```python
from build123d import *

# Parameters (mm, degrees)
SKETCH1_R           = 2.6
BOSS_EXTRUDE3_DEPTH = 10
SKETCH5_R           = 5
CUT_EXTRUDE3_DEPTH  = 20
FILLET2_R           = 1


with BuildPart() as part:
    # Sketch1 → Boss-Extrude3 (new body)
    with BuildSketch(Plane(origin=(0, 0, 0), x_dir=(1, 0, 0), z_dir=(0, 1, 0))):
        with BuildLine():
            Line((-13.5, -10), (13.5, -10))
            ThreePointArc((13.5, -10), (15.621320344, -9.121320344), (16.5, -7))
            Line((16.5, -7), (16.5, 7))
            ThreePointArc((16.5, 7), (15.621320344, 9.121320344), (13.5, 10))
            Line((13.5, 10), (-13.5, 10))
            ThreePointArc((-13.5, 10), (-15.621320344, 9.121320344), (-16.5, 7))
            Line((-16.5, 7), (-16.5, -7))
            ThreePointArc((-16.5, -7), (-15.621320344, -9.121320344), (-13.5, -10))
        make_face()
        with Locations((10.5, 0)):
            Circle(SKETCH1_R, mode=Mode.SUBTRACT)
        with Locations((-10.5, 0)):
            Circle(SKETCH1_R, mode=Mode.SUBTRACT)
    extrude(amount=BOSS_EXTRUDE3_DEPTH)

    # Sketch5 → Cut-Extrude3 (cut)
    with BuildSketch(Plane(origin=(0, 0, -10), x_dir=(-1, 0, 0), z_dir=(0, 0, -1))):
        with Locations((0, 10.2)):
            Circle(SKETCH5_R)
    extrude(amount=-CUT_EXTRUDE3_DEPTH, mode=Mode.SUBTRACT)

    # Fillet2
    fillet2_edges = [part.edges().sort_by_distance(p)[0] for p in [
        (0, 0, 10),
        (-15.621320344, 0, 9.121320344),
        (-16.5, 0, 0),
        (-15.621320344, 0, -9.121320344),
        (0, 0, -10),
        (15.621320344, 0, -9.121320344),
        (16.5, 0, 0),
        (15.621320344, 0, 9.121320344),
    ]]
    fillet(fillet2_edges, radius=FILLET2_R)


solid = part.part
```
Part model, mm, in its own coordinate system. Round coordinates to 2 decimals unless told otherwise and drop trailing zeros. Loops run counter-clockwise (first coordinate to the right, second up) from the corner with the lowest first, then second, coordinate; pieces in that order, holes last.
Item 1: Drill centre lines: line 1 (X direction, y = 5, z = 0); line 2 (Z direction, x = -10.5, y = 2.5); line 3 (X direction, y = 5.75, z = 0). Where is each one in solid material? Low to high.
Item 2: Cut at D-D, the plane y = 3.25. Give the cut face in (x, z), then the cut area to 3 significant figures.
Item 3: Drop a flat-ended pin along its axis: P1, Ø3, axis at x = 1.5, z = -0.5, coming from the +Y side. Give the stop position or say it passes through.
Item 4: Cut at A-A, the plane y = 9.5. Give the cut face in (x, z), then the cut area to 3 significant figures.
Item 5: Mould opens along Z. For faces 1 (the face through (11.9, 10, -2.4)), 2 (the face through (-0.189, 0.301, -9.715)), 3 (the face through (-8.02, 4.93, -0.78)) say: +Z half, -Z half, draft (parallel to the pull), parting line (faces both ways), or undercut.
Item 6: Cut at B-B, the plane x = 10.5. Give the cut face in (y, z), then the cut area to 3 significant figures.
A:
1. line 1: x = -16.5 to -13.1, -7.9 to 7.9, 13.1 to 16.5
1. line 2: z = -10 to -2.6, 2.6 to 10
1. line 3: x = -16.5 to -13.1, -7.9 to -2.28, 2.28 to 7.9, 13.1 to 16.5
2. outline: (-16.5, -7) arc R3 ccw to (-13.5, -10) - (13.5, -10) arc R3 ccw to (16.5, -7) - (16.5, 7) arc R3 ccw to (13.5, 10) - (-13.5, 10) arc R3 ccw to (-16.5, 7) - close; hole circle Ø5.2 at (-10.5, 0); hole circle Ø5.2 at (10.5, 0)
2. area: 610 mm2
3. P1: stops at y = 6.2
4. outline: (-16.5, -7) arc R3 ccw to (-13.5, -10) - (-4.95, -10) - (-4.95, 10) - (-13.5, 10) arc R3 ccw to (-16.5, 7) - close; (4.95, -10) - (13.5, -10) arc R3 ccw to (16.5, -7) - (16.5, 7) arc R3 ccw to (13.5, 10) - (4.95, 10) - close; hole circle Ø5.2 at (-10.5, 0); hole circle Ø5.2 at (10.5, 0)
4. area: 412 mm2
5. face 1: draft
5. face 2: -Z half
5. face 3: undercut
6. outline: (0, -9) arc R1 ccw to (1, -10) - (10, -10) - (10, -2.6) - (0, -2.6) - close; (0, 2.6) - (10, 2.6) - (10, 10) - (1, 10) arc R1 ccw to (0, 9) - close
6. area: 148 mm2
